Part model, mm, in its own coordinate system. Round coordinates to 2 decimals unless told otherwise and drop trailing zeros. Order: outer loops, then holes, each group sorted by start corner. A loop starts at its lowest first (then second) coordinate and runs counter-clockwise, first axis right, second up. Notation, with made-up numbers: (-23, -18.5) - (2, -18.5) arc R25 ccw to (2, 16.5) - close; hole circle Ø11 at (-39, 78). An arc over 180 degrees is marked (long way). Return JSON: item names as keys, results as strings. Group by question number.
Item 1: Saw through at C-C on y = 34. List the corners of the cut face in (x, z), and give its area (3 significant figures).
Item 2: Saw through at A-A on x = 31. List the corners of the cut face in (y, z).
Item 3: Drop flat-ended pins along their axis: pin 1 (8 mm diameter, centred on x = 39, y = 32, fed in from -Z); pin 2 (3 mm diameter, centred on x = 42.5, y = 31, fed in from -Z); pin 3 (4 mm diameter, centred on x = 2.5, z = 6, fed in from +Y). Give the stop position or say it passes through.
Item 4: Saw through at B-B on y = 16.5. List the corners of the cut face in (x, z), and give its area (3 significant figures).
Item 5: Probe probe 1 along X at (y, z) = (9.5, 0); probe 2 along Y at (x, z) = (11.5, 20.5); probe 3 along X at (y, z) = (3.5, -13.5). List the from-to ranges inside material, lowest first.
```python
from build123d import *

# Parameters (mm, degrees)
EXTRUDE1_DEPTH = 12
EXTRUDE2_DEPTH = 40
REVOLVE1_ANGLE = 180


with BuildPart() as part:
    # Sketch1 → Extrude1 (new body)
    with BuildSketch(Plane(origin=(0, 0, 0), x_dir=(1, 0, 0), z_dir=(0, 1, 0))):
        with BuildLine():
            Line((0, -22), (40, -22))
            Line((40, -22), (59.052558883, -11))
            Line((59.052558883, -11), (59.052558883, 11))
            Line((59.052558883, 11), (40, 22))
            Line((40, 22), (0, 22))
            ThreePointArc((0, 22), (-22, 0), (0, -22))
        make_face()
    extrude(amount=EXTRUDE1_DEPTH)

    # Sketch2 → Extrude2 (add)
    with BuildSketch(Plane(origin=(0, 0, 0), x_dir=(0, 0, -1), z_dir=(1, 0, 0))):
        Polygon((0, 40), (-22, 12), (22, 12), align=None)
    extrude(amount=EXTRUDE2_DEPTH)

    # Sketch3 → Revolve1 (revolve)
    with BuildSketch(Plane.ZY):
        Polygon((0, 40), (0, 12), (22, 12), align=None)
    revolve(axis=Axis((0, 40, 0), (0, -1, 0)), revolution_arc=REVOLVE1_ANGLE)

    # Sketch4 → Loft1 section 0
    with BuildSketch(Plane(origin=(0, 12, 0), x_dir=(-1, 0, 0), z_dir=(0, 1, 0)), mode=Mode.PRIVATE) as loft1_s0:
        Polygon((-59.052558883, 11), (-59.052558883, -11), (-40, -22), (-40, 22), align=None)
    loft([Vertex(40, 40, 0), loft1_s0.sketch])


solid = part.part
```
Filled in:
{
 "1": {"outline": "(0, -4.71) - (40, -4.71) - (44.08, -2.36) - (44.08, 2.36) - (40, 4.71) - (0, 4.71) arc R4.71 ccw to start", "area": "441 mm^2"},
 "2": {"outline": "(0, -22) - (12, -22) - (40, 0) - (12, 22) - (0, 22) - close"},
 "3": {"pin 1": "stops at z = -9.43", "pin 2": "stops at z = -7.09", "pin 3": "stops at y = 34.91"},
 "4": {"outline": "(0, -18.46) - (40, -18.46) - (55.99, -9.23) - (55.99, 9.23) - (40, 18.46) - (0, 18.46) arc R18.46 ccw to start", "area": "2,460 mm^2"},
 "5": {"probe 1": "x = -22 to 59.05", "probe 2": "y = 0 to 13.91", "probe 3": "x = -17.37 to 54.72"}
}
